```python
from build123d import *

# Parameters (mm, degrees)
F0_W     = 60
F0_H     = 50
F1_DEPTH = 8
F2_T     = -3
F3_R     = 3
F4_DEPTH = 6
F6_D     = 3
F6_DEPTH = 4
F6_TIP   = 0.9012909285
F7_W     = 60
F7_H     = 50
F8_DEPTH = 8


with BuildPart() as f1:
    # F0 (on Top) → F1 (new body)
    with BuildSketch(Plane.XY):
        Rectangle(F0_W, F0_H)
    extrude(amount=F1_DEPTH)

    # F2
    f2_openings = [f1.faces().sort_by_distance(p)[0] for p in [
        (0, 0, 8),
    ]]
    offset(amount=F2_T, openings=f2_openings)

    # F3 (on face) → F4 (join)
    with BuildSketch(Plane.XY):
        with Locations((-20.7, -16.75)):
            Circle(F3_R)
        with Locations((-20.7, 16.75)):
            Circle(F3_R)
        with Locations((23.8, -16.75)):
            Circle(F3_R)
        with Locations((23.8, 16.75)):
            Circle(F3_R)
    extrude(amount=F4_DEPTH)

    # F6
    with Locations(Plane.XY.offset(6)):
        with Locations((23.8, 16.75), (23.8, -16.75), (-20.7, -16.75), (-20.7, 16.75)):
            Hole(F6_D / 2, depth=F6_DEPTH)
            with Locations((0, 0, -(F6_DEPTH + F6_TIP / 2))):  # 118° drill point
                Cone(0, F6_D / 2, F6_TIP, mode=Mode.SUBTRACT)

    # F7 (on face) → F8 (join, through all)
    with BuildSketch(Plane.XY):
        with BuildLine():
            ThreePointArc((29.2079207921, 28.9207920792), (0, 26), (-29.2079207921, 28.9207920792))
            ThreePointArc((-29.2079207921, 28.9207920792), (-32.8837617935, 27.7719880805), (-33.8864353312, 24.0536277603))
            ThreePointArc((-33.8864353312, 24.0536277603), (-31, 0), (-33.8864353312, -24.0536277603))
            ThreePointArc((-33.8864353312, -24.0536277603), (-33.1452733553, -27.4712862077), (-30, -29))
            ThreePointArc((-30, -29), (-29.2382778582, -28.8471228354), (-28.475771577, -28.698206013))
            ThreePointArc((-28.475771577, -28.698206013), (0.379534182, -26.0011232313), (29.2130634934, -28.9218274993))
            ThreePointArc((29.2130634934, -28.9218274993), (32.8855788702, -27.7700964936), (33.8864353312, -24.0536277603))
            ThreePointArc((33.8864353312, -24.0536277603), (31.0022348413, -0.4407544994), (33.5761126117, 23.2079568676))
            ThreePointArc((33.5761126117, 23.2079568676), (33.7840774597, 24.1049195845), (34, 25))
            ThreePointArc((34, 25), (32.532951161, 28.0958291968), (29.2079207921, 28.9207920792))
        make_face()
        Rectangle(F7_W, F7_H, mode=Mode.SUBTRACT)
        with BuildLine():
            ThreePointArc((33.5761126117, 23.2079568676), (33.8925859301, 24.079253142), (34, 25))
            ThreePointArc((34, 25), (33.7840774597, 24.1049195845), (33.5761126117, 23.2079568676))
        make_face()
        with BuildLine():
            ThreePointArc((-28.475771577, -28.698206013), (-29.2382778582, -28.8471228354), (-30, -29))
            ThreePointArc((-30, -29), (-29.2230907556, -28.9238261972), (-28.475771577, -28.698206013))
        make_face()
    extrude(amount=F8_DEPTH)


solid = f1.part
```
Input: part model. Units: mm. Frame: model coordinates. A direction names the side the tool comes from. Coordinates: 2 decimals unless noted, no trailing zeros. Write each loop counter-clockwise with the first axis right and the second up, starting at its lowest first coordinate (ties: lowest second). Pieces come first, ordered by that corner, then holes.
1) Section A-A on z = 5. State how many separate pieces and enclosed holes the cut face has, and give its area (3 significant figures).
2) Material intervals for line 1 along Y through (x, z) = (23.8, 3.65); line 2 along Y through (x, z) = (-20.7, 4.75); line 3 along X through (y, z) = (-16.75, 3.7), sorted ascending.
3) Mould query, pull axis X, two halves, no side actions, for faces 3 (the cylindrical face through (-31, 0, 4)), 4 (the cylindrical face through (-20.505, 18.237, 3.972)), 5 (the cylindrical face through (31.005, -0.775, 3.944)). Classes: pulls with the +X half, pulls with the -X half, needs draft (parallel to the pull), parting line crosses it, or undercut.
4) Pin query (flat end, axial travel): pin 1 Ø3 at (x, y) = (-14, -10) entering from +Z; pin 2 Ø2.5 at (x, y) = (23.8, 16.75) entering from +Z; pin 3 Ø6.5 at (x, y) = (-21, -17.5) entering from +Z. Return the tip coordinate at first contact, or that it passes through.
5) Set-up query: faces 1 (the flat face through (0, 0, 0)), 2 (the flat face through (0, 0, 3)). Return all of +Z, -Z, +X, -X, +Y, -Y with unobstructed straight access to the full face (end or side cutting, diameter ignored); none if empty.
6) Section C-C on x = -3.5. Output: boundary loops of the cut face in (y, z).
7) Section B-B on x = 8.5. Output: boundary loops of the cut face in (y, z).
Check result:
1. separate pieces: 5
1. enclosed holes: 5
1. area: 1,200 mm2
2. line 1: y = -27.94 to -22, -19.75 to -18.25, -15.25 to -13.75, 13.75 to 15.25, 18.25 to 19.75, 22 to 27.93
2. line 2: y = -27.41 to -22, -19.75 to -18.25, -15.25 to -13.75, 13.75 to 15.25, 18.25 to 19.75, 22 to 27.46
2. line 3: x = -32.39 to -27, -23.7 to -22.2, -19.2 to -17.7, 20.8 to 22.3, 25.3 to 26.8, 27 to 32.4
3. face 3: pulls with the -X half
3. face 4: undercut
3. face 5: pulls with the +X half
4. pin 1: stops at z = 3
4. pin 2: stops at z = 1.85
4. pin 3: stops at z = 6
5. face 1: -Z, +X, -X, +Y, -Y
5. face 2: +Z
6. outline: (-26.04, 0) - (26.04, 0) - (26.04, 8) - (22, 8) - (22, 3) - (-22, 3) - (-22, 8) - (-26.04, 8) - close
7. outline: (-26.25, 0) - (26.25, 0) - (26.25, 8) - (22, 8) - (22, 3) - (-22, 3) - (-22, 8) - (-26.25, 8) - close
